Here's how the part is built. I have some questions about the finished solid (model axes, mm). Face numbers are marked on the shaded views. Coordinates: 2 decimals unless noted, no trailing zeros. Write each loop counter-clockwise with the first axis right and the second up, starting at its lowest first coordinate (ties: lowest second). Pieces come first, ordered by that corner, then holes.
Item 1: Please list where these lines run through material, in increasing order: line 1 (Z direction, x = 21.25, y = 15.25); line 2 (X direction, y = 18.5, z = -52.5); line 3 (X direction, y = 11.25, z = -32).
Item 2: I want a section at B-B (x = 21.25). Please give me the cut outline in (y, z), and give its area (3 significant figures).
Item 3: If we mould it in two halves opening along Z, with no side actions, what happens to the marked faces 1, 2, 3 and 4? For each: pulls with the +Z half, pulls with the -Z half, needs draft (parallel to the pull), parting line crosses it, or undercut.
Item 4: I want a section at D-D (z = 64.5). Please give me the cut outline in (x, y), and give its area (3 significant figures).
Item 5: I want a section at A-A (z = 9.5). Please give me the cut outline in (x, y).
Item 6: I want a section at C-C (y = 6). Count the separate pieces of the cut face and the enclosed holes in it, and give its area (3 significant figures).
Item 7: I'm going to push flat-ended pins straight in: P1, Ø5, axis at x = -27, z = 39.5, coming from the -Y side; P2, Ø24, axis at x = 21.25, z = -64.5, coming from the +Y side. Where does each tip first touch, or does it pass through?
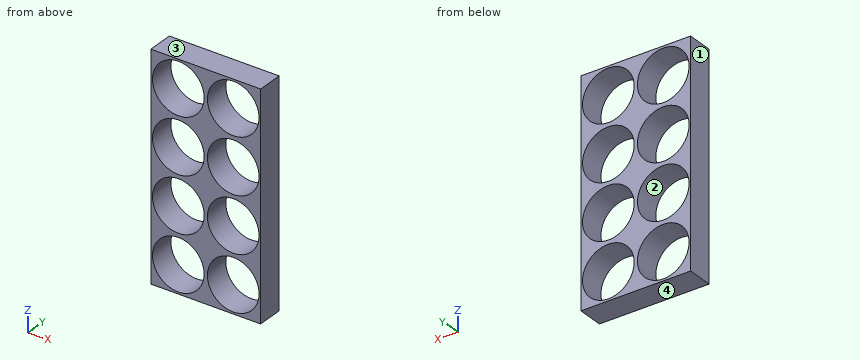
Autodesk Inventor part; units mm, degrees
ref_plane "YZ Plane" through (0, 0, 0) normal (1, 0, 0) x (0, 1, 0)
ref_plane "XZ Plane" through (0, 0, 0) normal (0, 1, 0) x (-1, 0, 0)
ref_plane "XY Plane" through (0, 0, 0) normal (0, 0, 1) x (1, 0, 0)
sketch "Sketch1" plane through (0, 0, 0) normal (0, 1, 0) x (-1, 0, 0)
  line L0 (42.5, 86) -> (-42.5, 86)
  line L1 (-42.5, 86) -> (-42.5, -86)
  line L2 (-42.5, -86) -> (42.5, -86)
  line L3 (42.5, -86) -> (42.5, 86)
  line L4 (42.5, 0) -> (-42.5, 0) construction
  circle A0 centre (21.25, 64.5) radius 20
  line L5 (-21.25, 86) -> (-21.25, -86) construction
  line L6 (21.25, -86) -> (21.25, 86) construction
  circle A1 centre (21.25, 21.5) radius 20
  circle A2 centre (21.25, -21.5) radius 20
  circle A3 centre (21.25, -64.5) radius 20
  circle A4 centre (-21.25, -64.5) radius 20
  circle A5 centre (-21.25, -21.5) radius 20
  circle A6 centre (-21.25, 21.5) radius 20
  circle A7 centre (-21.25, 64.5) radius 20
  line L7 (42.5, 64.5) -> (-42.5, 64.5) construction
  line L8 (42.5, 21.5) -> (-42.5, 21.5) construction
  line L9 (42.5, -21.5) -> (-42.5, -21.5) construction
  line L10 (42.5, -64.5) -> (-42.5, -64.5) construction
  point P0 (0, 0)
  point P1 (0, 0)
  dimension "d0" = 172
  dimension "d1" = 85
  dimension "d2" = 40
  dimension "d3" = 42.5
  dimension "d4" = 21.25
  dimension "d5" = 43
  dimension "d6" = 43
  dimension "d7" = 43
  dimension "d8" = 21.5
extrude "Extrusion1" add sketch "Sketch1" along normal blind 20
equation "\"d3\" = 0.5 * d1"
equation "\"d4\" = 0.25 * d1"
equation "\"d5\" = 0.25 * d0"
equation "\"d6\" = d5"
equation "\"d7\" = d5"
equation "\"d8\" = 0.125 * d0"
properties part number "Cell_Spacer" material "ABS Plastic"
Answer:
1. line 1: z = -86 to -84.5, -44.5 to -41.5, -1.5 to 1.5, 41.5 to 44.5, 84.5 to 86
1. line 2: x = -42.5 to -37.25, -5.25 to 5.25, 37.25 to 42.5
1. line 3: x = -42.5 to -38.27, -4.23 to 4.23, 38.27 to 42.5
2. outline: (0, -86) - (20, -86) - (20, -84.5) - (0, -84.5) - close; (0, -44.5) - (20, -44.5) - (20, -41.5) - (0, -41.5) - close; (0, -1.5) - (20, -1.5) - (20, 1.5) - (0, 1.5) - close; (0, 41.5) - (20, 41.5) - (20, 44.5) - (0, 44.5) - close; (0, 84.5) - (20, 84.5) - (20, 86) - (0, 86) - close
2. area: 240 mm2
3. face 1: needs draft
3. face 2: undercut
3. face 3: pulls with the +Z half
3. face 4: pulls with the -Z half
4. outline: (-42.5, 0) - (-41.25, 0) - (-41.25, 20) - (-42.5, 20) - close; (-1.25, 0) - (1.25, 0) - (1.25, 20) - (-1.25, 20) - close; (41.25, 0) - (42.5, 0) - (42.5, 20) - (41.25, 20) - close
4. area: 100 mm2
5. outline: (-42.5, 0) - (-37.25, 0) - (-37.25, 20) - (-42.5, 20) - close; (-5.25, 0) - (5.25, 0) - (5.25, 20) - (-5.25, 20) - close; (37.25, 0) - (42.5, 0) - (42.5, 20) - (37.25, 20) - close
6. separate pieces: 1
6. enclosed holes: 8
6. area: 4,570 mm2
7. P1: stops at y = 0
7. P2: passes through
